```python
from build123d import *

# Parameters (mm, degrees)
SKETCH_R      = 1.5
PAD_DEPTH     = 40
SKETCH001_W   = 10
SKETCH001_H   = 37
SKETCH001_W_2 = 40
POCKET_DEPTH  = 31.890025


with BuildPart() as part:
    # Sketch → Pad (new body)
    with BuildSketch(Plane.XY):
        with BuildLine():
            Line((0, 25), (19.905684, 25))
            ThreePointArc((46.094316, 25), (33, 31.889025), (19.905684, 25))
            Line((66, 25), (46.094316, 25))
            Line((66, 0), (66, 25))
            Line((0, 0), (66, 0))
            Line((0, 25), (0, 0))
        make_face()
        with Locations((33, 28.6)):
            Circle(SKETCH_R, mode=Mode.SUBTRACT)
        with Locations((43.91192, 9.7)):
            Circle(SKETCH_R, mode=Mode.SUBTRACT)
        with Locations((22.08808, 9.7)):
            Circle(SKETCH_R, mode=Mode.SUBTRACT)
        with Locations((4, 19)):
            Circle(SKETCH_R, mode=Mode.SUBTRACT)
        with Locations((4, 6)):
            Circle(SKETCH_R, mode=Mode.SUBTRACT)
        with Locations((62, 19)):
            Circle(SKETCH_R, mode=Mode.SUBTRACT)
        with Locations((62, 6)):
            Circle(SKETCH_R, mode=Mode.SUBTRACT)
    extrude(amount=PAD_DEPTH)

    # Sketch001 → Pocket (cut, through all)
    with BuildSketch(Plane.XZ):
        with Locations((5, 21.5)):
            Rectangle(SKETCH001_W, SKETCH001_H)
        with Locations((33, 18.5)):
            Rectangle(SKETCH001_W_2, SKETCH001_H)
        with Locations((61, 21.5)):
            Rectangle(SKETCH001_W, SKETCH001_H)
    extrude(amount=-POCKET_DEPTH, mode=Mode.SUBTRACT)


solid = part.part
```
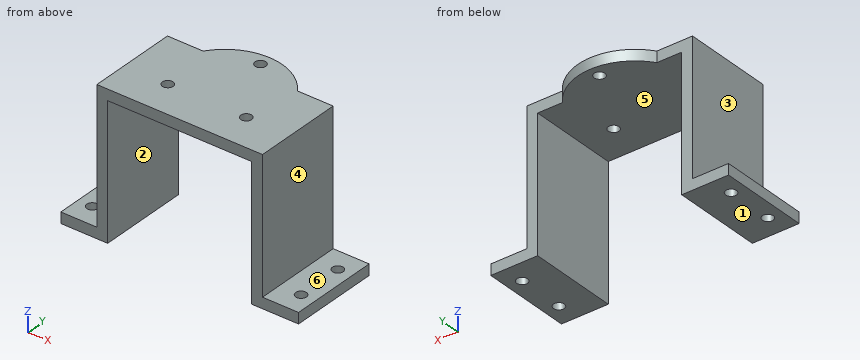
Source: CAD feature listing. Evaluate the final solid. Frame: model axes, mm. Face numbers are marked on the shaded views. A direction names the side the tool comes from. Round coordinates to 2 decimals unless told otherwise and drop trailing zeros. Loops run counter-clockwise (first coordinate to the right, second up) from the corner with the lowest first, then second, coordinate; pieces in that order, holes last.
1. Contact query for flat-ended pins moving along their axis: pin 1 (5 mm diameter, centred on x = 4, y = 19, fed in from +Z); pin 2 (7.5 mm diameter, centred on y = 11, z = 13, fed in from -X); pin 3 (1 mm diameter, centred on x = 11, z = 32, fed in from +Y). Output: stop coordinate, or through.
2. Section query A-A on z = 5.5. Output: boundary loops of the cut face in (x, y).
3. Ray query, L1, parallel to Y at x = 62, z = 1.85; L2, parallel to X at y = 6, z = 1.85; L3, parallel to X at y = 17, z = 32.5. Return the intervals inside material, ascending.
4. Section query B-B on x = 33. Output: boundary loops of the cut face in (y, z), and give its area (3 significant figures).
5. Access query for the marked faces 1 and 2. Directions: +Z, -Z, +X, -X, +Y, -Y. A direction counts if a zero-diameter tool reaches every point of the face in a straight line with its end or side. Return the directions, or none.
6. Section query C-C on y = 19. Output: boundary loops of the cut face in (x, z).
7. Mould query, pull axis X, two halves, no side actions, for the marked faces 3, 4, 5 and 6. Classes: released by +X, released by -X, zero draft, split by the parting line, or undercut.
8. Section query D-D on x = 62. Output: boundary loops of the cut face in (y, z), and give its area (3 significant figures).
Answers below:
1. pin 1: stops at z = 3
1. pin 2: stops at x = 10
1. pin 3: stops at y = 25
2. outline: (10, 0) - (13, 0) - (13, 25) - (10, 25) - close; (53, 0) - (56, 0) - (56, 25) - (53, 25) - close
3. L1: y = 0 to 4.5, 7.5 to 17.5, 20.5 to 25
3. L2: x = 0 to 2.5, 5.5 to 13, 53 to 60.5, 63.5 to 66
3. L3: x = 10 to 13, 53 to 56
4. outline: (0, 37) - (27.1, 37) - (27.1, 40) - (0, 40) - close; (30.1, 37) - (31.89, 37) - (31.89, 40) - (30.1, 40) - close
4. area: 86.7 mm2
5. face 1: -Z, +X, -X, +Y, -Y
5. face 2: -Z, +Y, -Y
6. outline: (0, 0) - (2.5, 0) - (2.5, 3) - (0, 3) - close; (5.5, 0) - (13, 0) - (13, 37) - (53, 37) - (53, 0) - (60.5, 0) - (60.5, 3) - (56, 3) - (56, 40) - (10, 40) - (10, 3) - (5.5, 3) - close; (63.5, 0) - (66, 0) - (66, 3) - (63.5, 3) - close
7. face 3: released by -X
7. face 4: released by +X
7. face 5: undercut
7. face 6: zero draft
8. outline: (0, 0) - (4.5, 0) - (4.5, 3) - (0, 3) - close; (7.5, 0) - (17.5, 0) - (17.5, 3) - (7.5, 3) - close; (20.5, 0) - (25, 0) - (25, 3) - (20.5, 3) - close
8. area: 57.0 mm2
